Autodesk Inventor part; units mm, degrees
ref_plane "YZ Plane" through (0, 0, 0) normal (1, 0, 0) x (0, 1, 0)
ref_plane "XZ Plane" through (0, 0, 0) normal (0, 1, 0) x (-1, 0, 0)
ref_plane "XY Plane" through (0, 0, 0) normal (0, 0, 1) x (1, 0, 0)
sketch "Sketch1" plane through (0, 0, 0) normal (0, 1, 0) x (-1, 0, 0)
  circle A0 centre (3.5103, 7.6377) radius 2.5797
  point P0 (0, 0)
  dimension "d0" = 5.1594
extrude "Extrusion1" add sketch "Sketch1" along normal blind 50.8
sketch "Sketch2" plane through (-3.5103, 50.8, 7.6377) normal (0, 1, 0) x (1, 0, 0)
  circle A0 centre (0, 0) radius 3.175
  point P0 (3.5103, 7.6377)
  dimension "d3" = 6.35
extrude "Extrusion2" add sketch "Sketch2" along normal blind 5.08
sketch "Sketch3" plane through (-3.5103, 55.88, 7.6377) normal (0, 1, 0) x (1, 0, 0)
  circle A0 centre (0, 0) radius 2.5797
  line L0 (2.231, 1.2951) -> (2.2371, -1.2846)
  line L1 (2.2371, -1.2846) -> (0.006, -2.5797)
  line L2 (0.006, -2.5797) -> (-2.231, -1.2951)
  line L3 (-2.231, -1.2951) -> (-2.2371, 1.2846)
  line L4 (-2.2371, 1.2846) -> (-0.006, 2.5797)
  line L5 (-0.006, 2.5797) -> (2.231, 1.2951)
  point P0 (3.5103, 7.6377)
extrude "Extrusion3" cut sketch "Sketch3" against normal blind 3.81 contours L0 L1 L2 L3 L4 L5
properties part number "Bolt 13_64 Representation"
Work out the finished part from the listing and answer in its coordinate system (mm). A direction names the side the tool comes from. Coordinates: 2 decimals unless noted, no trailing zeros. Order: outer loops, then holes, each group sorted by start corner. A loop starts at its lowest first (then second) coordinate and runs counter-clockwise, first axis right, second up. Notation, with made-up numbers: (53.25, 68.5) - (66.25, 68.5) arc R16 ccw to (66.25, 82.5) - close; hole circle Ø1 at (54.25, 62). An arc over 180 degrees is marked (long way). Answer as a JSON object with one key per item and string values.
1. Find section C-C on y = 36.5. Determine the outline of the cut face in (x, z).
Output values:
{"outline": "circle Ø5.16 at (-3.51, 7.64)"}
2. Find section A-A on x = -2.5. Determine the outline of the cut face in (y, z), plus the area to 3 significant figures.
Output values:
{"outline": "(0, 5.26) - (50.8, 5.26) - (50.8, 4.63) - (55.88, 4.63) - (55.88, 5.64) - (52.07, 5.64) - (52.07, 9.63) - (55.88, 9.63) - (55.88, 10.65) - (50.8, 10.65) - (50.8, 10.01) - (0, 10.01) - close", "area": "257 mm²"}
3. Find section B-B on z = 9.75. Determine the outline of the cut face in (x, y), plus the area to 3 significant figures.
Output values:
{"outline": "(-5.88, 50.8) - (-4.99, 50.8) - (-4.99, 0) - (-2.03, 0) - (-2.03, 50.8) - (-1.14, 50.8) - (-1.14, 55.88) - (-2.7, 55.88) - (-2.7, 52.07) - (-4.32, 52.07) - (-4.32, 55.88) - (-5.88, 55.88) - close", "area": "168 mm²"}
4. A tool of negligible diameter and unlimited length cuts with its end or side. For faces 5 (the face through (-2, 55.88, 10)), 6 (the face through (-2.4, 54, 5.7)), from which of +Z, -Z, +X, -X, +Y, -Y can it reach the whole face along a straight path? Write none if from no direction.
Output values:
{"face 5": "+Z, -Z, +X, -X, +Y", "face 6": "+Y"}
5. The mould has two halves that part along X. Classify faces 1 (the face through (-1, 50.8, 6)), 2 (the face through (-4, 52.07, 8)), 3 (the face through (-4.897, 25.044, 5.462)), 4 (the face through (-2.37, 54, 9.56)): +X half, -X half, draft (parallel to the pull), parting line (faces both ways), or undercut.
Output values:
{"face 1": "draft", "face 2": "undercut", "face 3": "parting line", "face 4": "undercut"}
6. Consider line 1 (Z direction, x = -3.75, y = 51); line 2 (Z direction, x = -5.75, y = 21); line 3 (Y direction, x = -3.75, z = 9.75). Determine where each line is inside the solid, lowest interval first.
Output values:
{"line 1": "z = 4.47 to 10.8", "line 2": "z = 6.36 to 8.92", "line 3": "y = 0 to 52.07"}
7. Each of these flat-tipped pins is pushed along its axis until it touches: P1, Ø2, axis at x = -1, y = 32, coming from the +Z side; P2, Ø3, axis at y = 33, z = 8, coming from the +X side; P3, Ø1.5, axis at x = -5.5, y = 39, coming from the +Z side. Where does it stop, or does it pass through?
Output values:
{"P1": "stops at z = 9.73", "P2": "stops at x = -0.93", "P3": "stops at z = 9.9"}
